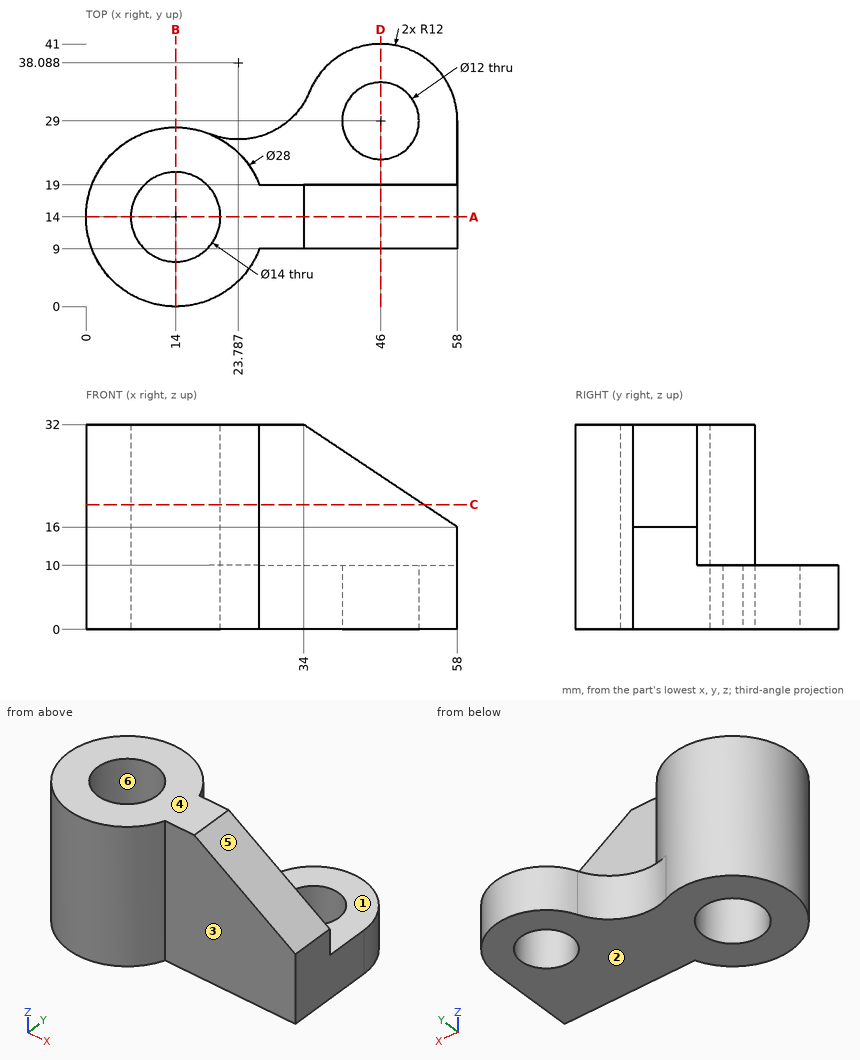
For this review, use the dimensioned drawing (mm, ordinates from the lowest corner) and the shaded views. A direction names the side the tool comes from. Give positions to 0.01 mm unless a question says otherwise; leave off trailing zeros. Loops run counter-clockwise (first coordinate to the right, second up) from the corner with the lowest first, then second, coordinate; pieces in that order, holes last.
Item 1: Insertion check: pin 1 (9.5 mm diameter, centred on x = 48, z = 14.5, fed in from -Y); pin 2 (4 mm diameter, centred on y = 11.5, z = 21.5, fed in from +X); pin 3 (5 mm diameter, centred on x = 15.5, z = 26.5, fed in from +Y). Each pin has a flat end and moves straight along its axis. Give the tip position at first contact, or say it passes through.
Item 2: Take a section at B-B, the plane x = 14. State the section outline as (y, z) points, and give its area (3 significant figures).
Item 3: For line 1 along Y through (x, z) = (14, 8); line 2 along Y through (x, z) = (46, 5.25); line 3 along Z through (x, y) = (33, 26.5), list the stretches that pass through material, from the lowest coordinate up.
Item 4: Take a section at C-C, the plane z = 19.5. State the section outline as (x, y) points, and give its area (3 significant figures).
Item 5: Take a section at D-D, the plane x = 46. State the section outline as (y, z) points, and give its area (3 significant figures).
Item 6: Draft analysis for pull direction X (two halves, no side actions). For the marked faces 4, 5 and 6, state which applies: +X half, -X half, draft (parallel to the pull), parting line (faces both ways), or undercut.
Item 7: Take a section at A-A, the plane y = 14. State the section outline as (x, z) points, and give its area (3 significant figures).
Item 8: Tool access review of the marked faces 1, 2 and 3: name each direction out of +Z, -Z, +X, -X, +Y, -Y from which nothing blocks a thin tool from reaching the whole face with its end or side.
Calculated:
1. pin 1: stops at y = 9
1. pin 2: stops at x = 52.75
1. pin 3: stops at y = 28
2. outline: (0, 0) - (7, 0) - (7, 32) - (0, 32) - close; (21, 0) - (28, 0) - (28, 32) - (21, 32) - close
2. area: 448 mm2
3. line 1: y = 0 to 7, 21 to 28
3. line 2: y = 9 to 23, 35 to 41
3. line 3: z = 0 to 10
4. outline: (27.08, 9) - (52.75, 9) - (52.75, 19) - (27.08, 19) arc R14 ccw (long way) to start; hole circle Ø14 at (14, 14)
4. area: 712 mm2
5. outline: (9, 0) - (23, 0) - (23, 10) - (19, 10) - (19, 24) - (9, 24) - close; (35, 0) - (41, 0) - (41, 10) - (35, 10) - close
5. area: 340 mm2
6. face 4: draft
6. face 5: +X half
6. face 6: undercut
7. outline: (0, 0) - (7, 0) - (7, 32) - (0, 32) - close; (21, 0) - (58, 0) - (58, 16) - (34, 32) - (21, 32) - close
7. area: 1,220 mm2
8. face 1: +Z, +X, +Y
8. face 2: -Z, +X, -X, +Y, -Y
8. face 3: +Z, -Z, +X, -Y
